from build123d import *

# Parameters (mm, degrees)
F0_W     = 762
F0_H     = 76.2
F1_DEPTH = 1270
F2_R     = 12.7
F2_R_2   = 38.1
F3_DEPTH = 25.4
F5_DEPTH = 1270.001
F6_R     = 19.05
F7_DEPTH = 1270.001


with BuildPart() as f1:
    # F0 (on Front) → F1 (new body)
    with BuildSketch(Plane.XZ):
        Rectangle(F0_W, F0_H)
    extrude(amount=F1_DEPTH)

    # F2 (on face) → F3 (cut)
    with BuildSketch(Plane(origin=(0, 0, -38.1), x_dir=(1, 0, 0), z_dir=(0, 0, -1))):
        with Locations((0, 1231.9)):
            Circle(F2_R)
        with Locations((0, 38.1)):
            Circle(F2_R)
        with Locations((0, 876.3)):
            Circle(F2_R_2)
        with Locations((0, 393.7)):
            Circle(F2_R_2)
    extrude(amount=-F3_DEPTH, mode=Mode.SUBTRACT)

    # F4 (on face) → F5 (cut, through all)
    with BuildSketch(Plane.XZ.offset(1270)):
        with BuildLine():
            Line((-381, -38.1), (381, -38.1))
            ThreePointArc((381, -38.1), (0, 10.991921), (-381, -38.1))
        make_face()
    extrude(amount=-F5_DEPTH, mode=Mode.SUBTRACT)

    # F6 (on face) → F7 (cut, through all)
    with BuildSketch(Plane(origin=(0, 0, 0), x_dir=(-1, 0, 0), z_dir=(0, 1, 0))):
        with Locations((-381, 38.1)):
            Circle(F6_R)
        with Locations((381, 38.1)):
            Circle(F6_R)
    extrude(amount=-F7_DEPTH, mode=Mode.SUBTRACT)


solid = f1.part
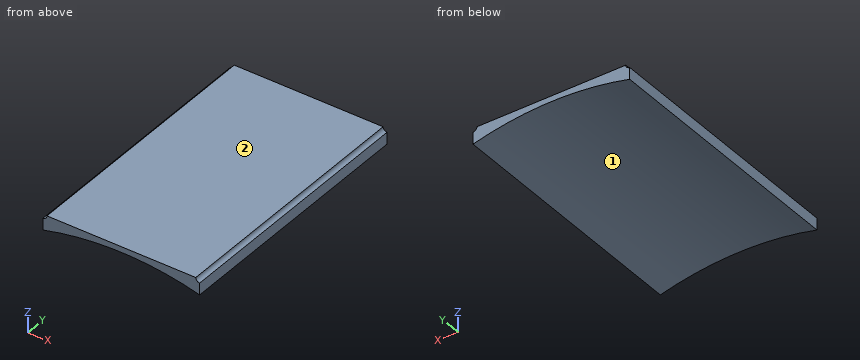
Part model, mm, in its own coordinate system. Face numbers are marked on the shaded views. Round coordinates to 2 decimals unless told otherwise and drop trailing zeros. Write each loop counter-clockwise with the first axis right and the second up, starting at its lowest first coordinate (ties: lowest second). Pieces come first, ordered by that corner, then holes. Notation, with made-up numbers: M 29.25,78.25 L 37.25,78.25 A19 ccw 37.25,102.25 Z; hole C 55.25,0 d5. An arc over 180 degrees is marked long. Return JSON: item names as keys, results as strings. Group by question number.
(1) Drill centre lines: probe 1 along Z at (x, y) = (-20.5, -388); probe 2 along Z at (x, y) = (40, -876); probe 3 along X at (y, z) = (-846, 33.5). Where is each one in solid material? Low to high.
(2) Saw through at A-A on z = -15.5. Write the cut outline in (x, y).
(3) Two-plate mould, pull along X, no slides. Class the marked faces 1 and 2: +X half, -X half, draft (parallel to the pull), parting line (faces both ways), or undercut.
(4) Pin check, flat tips, straight feed: pin 1 Ø4 at (x, z) = (149.5, 1) entering from -Y; pin 2 Ø2 at (x, y) = (175, -987.5) entering from -Z. Stop position of each tip, or through.
(5) Saw through at C-C on x = -177. Write the cut outline in (y, z).
(6) Saw through at B-B on y = -1042.5. Write the cut outline in (x, z).
(7) Saw through at D-D on x = 5. Write the cut outline in (y, z), then the cut area to 3 significant figures.
Returned:
{
 "1": {"probe 1": "10.85 to 38.1", "probe 2": "10.46 to 38.1", "probe 3": "-362.51 to 362.51"},
 "2": {"outline": "M -381,-1270 L -280.95,-1270 L -280.95,0 L -381,0 Z; M 280.95,-1270 L 381,-1270 L 381,0 L 280.95,0 Z"},
 "3": {"face 1": "undercut", "face 2": "draft"},
 "4": {"pin 1": "through", "pin 2": "z = 0.65"},
 "5": {"outline": "M -1270,0.53 L 0,0.53 L 0,38.1 L -1270,38.1 Z"},
 "6": {"outline": "M -381,-38.1 A1503.01 cw 381,-38.1 L 381,19.05 A19.05 cw 361.95,38.1 L -361.95,38.1 A19.05 cw -381,19.05 Z"},
 "7": {"outline": "M -1270,10.98 L 0,10.98 L 0,38.1 L -1270,38.1 Z", "area": "34,400 mm²"}
}
